from build123d import *

# Parameters (mm, degrees)
SKETCH_1_R          = 2.594697184
SKETCH_1_W          = 50.755093491
SKETCH_1_H          = 34.509114599
EXTRUDE_1_DEPTH     = 5
SKETCH_2_W          = 12.017165499
SKETCH_2_H          = 2.614231611
CUT_EXTRUDE_1_DEPTH = 10
SKETCH_3_W          = 7.527857493
SKETCH_3_H          = 30.984988894
CUT_EXTRUDE_2_DEPTH = 3
SKETCH_4_W          = 11.818287361
SKETCH_4_H          = 34.509114599
CUT_EXTRUDE_3_DEPTH = 10
SKETCH_5_W          = 8.407446584
SKETCH_5_H          = 13.753485989
CUT_EXTRUDE_4_DEPTH = 3
SKETCH_6_W          = 45.235718037
SKETCH_6_H          = 4.020952714
CUT_EXTRUDE_5_DEPTH = 10


with BuildPart() as part:
    # 草图1 → 凸台-拉伸1 (new body)
    with BuildSketch(Plane.XY):
        with BuildLine():
            Line((-33.053422138, 25.444897132), (26.761429335, 25.444897132))
            ThreePointArc((26.761429335, 25.444897132), (28.882749679, 24.566217475), (29.761429335, 22.444897132))
            Line((29.761429335, 22.444897132), (29.761429335, -19.896984924))
            ThreePointArc((29.761429335, -19.896984924), (28.882749679, -22.018305267), (26.761429335, -22.896984924))
            Line((26.761429335, -22.896984924), (-33.053422138, -22.896984924))
            ThreePointArc((-33.053422138, -22.896984924), (-35.174742482, -22.018305267), (-36.053422138, -19.896984924))
            Line((-36.053422138, -19.896984924), (-36.053422138, 22.444897132))
            ThreePointArc((-36.053422138, 22.444897132), (-35.174742482, 24.566217475), (-33.053422138, 25.444897132))
        make_face()
        with Locations((-30.585365854, 20.792682927)):
            Circle(SKETCH_1_R, mode=Mode.SUBTRACT)
        with Locations((24.414634146, 20.792682927)):
            Circle(SKETCH_1_R, mode=Mode.SUBTRACT)
        with Locations((-30.585365854, -17.907317073)):
            Circle(SKETCH_1_R, mode=Mode.SUBTRACT)
        with Locations((24.414634146, -17.907317073)):
            Circle(SKETCH_1_R, mode=Mode.SUBTRACT)
        with Locations((-3.1480179, 1.476070041)):
            Rectangle(SKETCH_1_W, SKETCH_1_H, mode=Mode.SUBTRACT)
    extrude(amount=EXTRUDE_1_DEPTH)

    # 草图2 → 切除-拉伸1 (cut)
    with BuildSketch(Plane.XZ.offset(22.896984924)):
        with Locations((-23.547762162, 1.307115806)):
            Rectangle(SKETCH_2_W, SKETCH_2_H)
    extrude(amount=-CUT_EXTRUDE_1_DEPTH, mode=Mode.SUBTRACT)

    # 草图3 → 切除-拉伸2 (cut)
    with BuildSketch(Plane(origin=(0, 0, 0), x_dir=(-1, 0, 0), z_dir=(0, 0, -1))):
        with Locations((32.289493392, 1.687877711)):
            Rectangle(SKETCH_3_W, SKETCH_3_H)
    extrude(amount=-CUT_EXTRUDE_2_DEPTH, mode=Mode.SUBTRACT)

    # 草图4 → 切除-拉伸3 (cut)
    with BuildSketch(Plane.XY.offset(5)):
        with Locations((28.138672527, 1.476070041)):
            Rectangle(SKETCH_4_W, SKETCH_4_H)
    extrude(amount=-CUT_EXTRUDE_3_DEPTH, mode=Mode.SUBTRACT)

    # 草图5 → 切除-拉伸4 (cut)
    with BuildSketch(Plane(origin=(0, 0, 0), x_dir=(-1, 0, 0), z_dir=(0, 0, -1))):
        with Locations((-11.110108677, 20.556252076)):
            Rectangle(SKETCH_5_W, SKETCH_5_H)
    extrude(amount=-CUT_EXTRUDE_4_DEPTH, mode=Mode.SUBTRACT)

    # 草图6 → 切除-拉伸5 (cut)
    with BuildSketch(Plane(origin=(0, 0, 0), x_dir=(-1, 0, 0), z_dir=(0, 0, -1))):
        with Locations((3.557230201, 19.345396997)):
            Rectangle(SKETCH_6_W, SKETCH_6_H)
    extrude(amount=-CUT_EXTRUDE_5_DEPTH, mode=Mode.SUBTRACT)


solid = part.part
Design review of the part built by this model. Coordinates are the model's own, in mm. A direction names the side the tool comes from. Give positions to 0.01 mm unless a question says otherwise; leave off trailing zeros. Order: outer loops, then holes, each group sorted by start corner. A loop starts at its lowest first (then second) coordinate and runs counter-clockwise, first axis right, second up.
1. Mouldability with a two-part tool opening along X and no side actions: class faces 5 (the flat face through (-17.539, -19, 1)), 6 (the cylindrical face through (-35.2, 24.54, 2.46)), 7 (the flat face through (-3, -22.897, 2)), 8 (the flat face through (19.061, 20, 2)) as +X half, -X half, draft (parallel to the pull), parting line (faces both ways), or undercut.
Solution:
face 5: undercut
face 6: -X half
face 7: draft
face 8: undercut
2. For pin 1 Ø0.5 at (y, z) = (-14.5, 0.5) entering from +X; pin 2 Ø1 at (y, z) = (15, 3) entering from +X; pin 3 Ø3.5 at (x, y) = (12, 24) entering from -Z, all flat-tipped, find the tip position at first contact; note any pin that passes through.
Solution:
pin 1: stops at x = -29.56
pin 2: stops at x = -28.53
pin 3: stops at z = 3
3. Add section C-C, the plane y = 5.5. State the section outline as (x, z) points, then the cut area to 3 significant figures.
Solution:
outline: (-36.05, 3) - (-28.53, 3) - (-28.53, 5) - (-36.05, 5) - close
area: 15.1 mm2
4. To check wall thickness, follow L1, parallel to Y at x = -21.5, z = 3.1; L2, parallel to Y at x = -22, z = 1; L3, parallel to Y at x = -27, z = 2.5. State the ranges of each line that lie inside material, in increasing order.
Solution:
L1: y = -22.9 to -15.78, 21.36 to 25.44
L2: y = 21.36 to 25.44
L3: y = 18.73 to 25.44
5. Tool access review of faces 1 (the flat face through (-26.175, 20, 2)), 2 (the flat face through (-32, -13.805, 1)), 3 (the flat face through (21, 18.731, 2)), 4 (the flat face through (11, 23, 3)): name each direction out of +Z, -Z, +X, -X, +Y, -Y from which nothing blocks a thin tool from reaching the whole face with its end or side.
Solution:
face 1: +Z, -Z
face 2: -Z, +X, -X
face 3: +Z, -Z, +X
face 4: -Z, +Y
6. Add section A-A, the plane x = 11. State the section outline as (y, z) points.
Solution:
outline: (-22.9, 0) - (-15.78, 0) - (-15.78, 5) - (-22.9, 5) - close; (21.36, 3) - (25.44, 3) - (25.44, 5) - (21.36, 5) - close
7. Add section B-B, the plane x = 20. State the section outline as (y, z) points, then the cut area to 3 significant figures.
Solution:
outline: (-22.9, 0) - (-15.78, 0) - (-15.78, 5) - (-22.9, 5) - close; (18.73, 0) - (25.44, 0) - (25.44, 5) - (18.73, 5) - close
area: 69.2 mm2
